Work out the finished part from the listing and answer in its coordinate system (mm). A direction names the side the tool comes from. Round coordinates to 2 decimals unless told otherwise and drop trailing zeros. Order: outer loops, then holes, each group sorted by start corner. A loop starts at its lowest first (then second) coordinate and runs counter-clockwise, first axis right, second up. Notation, with made-up numbers: (42.5, 32.25) -> (59.5, 32.25) arc R22 ccw to (59.5, 38.25) -> close; hole circle Ø5 at (-10.75, -13.75). An arc over 180 degrees is marked (long way). Use one line per item in the form item = value.
```python
from build123d import *

# Parameters (mm, degrees)
F0_W     = 5
F0_H     = 4
F1_DEPTH = 5
F2_R     = 1.99999
F3_R     = 1
F4_DEPTH = 25
F7_W     = 3
F7_H     = 4
F8_DEPTH = 4


# Not quite as in the source:
# - a fillet or chamfer is up to 0.001 mm smaller than in the source, because OpenCascade refuses the exact size


with BuildPart() as f1:
    # F0 (on Top) → F1 (new body)
    with BuildSketch(Plane.XY):
        with Locations((2.5, 2)):
            Rectangle(F0_W, F0_H)
    extrude(amount=F1_DEPTH)

    # F2 (radius 2 in the source; OpenCascade refuses exactly that, so slightly less here)
    f2_edges = [f1.edges().sort_by_distance(p)[0] for p in [
        (2.5, 0, 5),
        (2.5, 4, 5),
    ]]
    fillet(f2_edges, radius=F2_R)

    # F3 (on face) → F4 (cut)
    with BuildSketch(Plane.YZ.offset(5)):
        with Locations((2, 3)):
            Circle(F3_R)
    extrude(amount=-F4_DEPTH, mode=Mode.SUBTRACT)

    # F7 (on face) → F8 (cut)
    with BuildSketch(Plane.XY.offset(5)):
        with Locations((2.5, 2)):
            Rectangle(F7_W, F7_H)
    extrude(amount=-F8_DEPTH, mode=Mode.SUBTRACT)


solid = f1.part
```
Item 1: Determine the mould class of faces 3 (the flat face through (2, 2, 1)), 4 (the flat face through (0, 2.4, 1.9)), 5 (the flat face through (5, 2.4, 1.9)), 6 (the cylindrical face through (4.507, 1.263, 3.676)) for opening direction X: released by +X, released by -X, zero draft, split by the parting line, or undercut.
Findings:
face_3 = undercut
face_4 = released by -X
face_5 = released by +X
face_6 = zero draft
Item 2: The part is cut by section A-A, the plane z = 1.25. Give the vertices of the cut face in (x, y).
Findings:
outline = (0, 0) -> (1, 0) -> (1, 4) -> (0, 4) -> close; (4, 0) -> (5, 0) -> (5, 4) -> (4, 4) -> close
Item 3: The part is cut by section C-C, the plane z = 3.85. Give the vertices of the cut face in (x, y), and give its area (3 significant figures).
Findings:
outline = (0, 0.19) -> (1, 0.19) -> (1, 1.47) -> (0, 1.47) -> close; (0, 2.53) -> (1, 2.53) -> (1, 3.81) -> (0, 3.81) -> close; (4, 0.19) -> (5, 0.19) -> (5, 1.47) -> (4, 1.47) -> close; (4, 2.53) -> (5, 2.53) -> (5, 3.81) -> (4, 3.81) -> close
area = 5.13 mm^2
Item 4: For faces 1 (the cylindrical face through (4.51, 0.57, 4.4)), 2 (the flat face through (1, 2, 1.7)), determine the directions among +Z, -Z, +X, -X, +Y, -Y from which every point of the face is accessible in a straight line to the end or side of a thin tool.
Findings:
face_1 = +Z, +X, -X, -Y
face_2 = +Z, +Y, -Y
Item 5: Consider line 1 along X through (y, z) = (1, 4); line 2 along Z through (x, y) = (4.3, 2); line 3 along Y through (x, z) = (0.4, 3.05). Determine where each line is inside the solid, lowest interval first.
Findings:
line_1 = 0 to 1, 4 to 5
line_2 = 0 to 2, 4 to 5
line_3 = 0 to 1, 3 to 4
Item 6: The part is cut by section D-D, the plane y = 2.25. Give the vertices of the cut face in (x, z).
Findings:
outline = (0, 0) -> (5, 0) -> (5, 2.03) -> (4, 2.03) -> (4, 1) -> (1, 1) -> (1, 2.03) -> (0, 2.03) -> close; (0, 3.97) -> (1, 3.97) -> (1, 4.98) -> (0, 4.98) -> close; (4, 3.97) -> (5, 3.97) -> (5, 4.98) -> (4, 4.98) -> close
Item 7: The part is cut by section B-B, the plane y = 3.2. Give the vertices of the cut face in (x, z).
Findings:
outline = (0, 0) -> (5, 0) -> (5, 4.6) -> (4, 4.6) -> (4, 1) -> (1, 1) -> (1, 4.6) -> (0, 4.6) -> close
